```python
from build123d import *

# Parameters (mm, degrees)
SKETCH_1_W          = 60
SKETCH_1_H          = 45
EXTRUDE_1_DEPTH     = 30
SKETCH_3_W          = 35.871207779
SKETCH_3_H          = 20
CUT_EXTRUDE_3_DEPTH = 62.71805709
CHAMFER_1_SIZE      = 8


with BuildPart() as part:
    # Эскиз1 → Вытянуть1 (new body)
    with BuildSketch(Plane(origin=(0, 0, 0), x_dir=(1, 0, 0), z_dir=(0, 1, 0))):
        with Locations((-19.019063342, 0)):
            Rectangle(SKETCH_1_W, SKETCH_1_H)
    extrude(amount=EXTRUDE_1_DEPTH)

    # Эскиз3 → Вытянуть3 (cut, through all)
    with BuildSketch(Plane(origin=(0, 30, 0), x_dir=(1, 0, 0), z_dir=(0, 1, 0))):
        with Locations((-38.69487705, 0)):
            Rectangle(SKETCH_3_W, SKETCH_3_H)
    extrude(amount=-CUT_EXTRUDE_3_DEPTH, mode=Mode.SUBTRACT)

    # Фаска1
    chamfer_1_edges = [part.edges().sort_by_distance(p)[0] for p in [
        (-49.019063342, 30, -16.25),
        (-49.019063342, 0, 16.25),
        (-49.019063342, 30, 16.25),
        (-49.019063342, 0, -16.25),
    ]]
    chamfer(chamfer_1_edges, length=CHAMFER_1_SIZE)


solid = part.part
```
Check sheet for the modelled part. Datum: model origin and axes. Units: mm. A direction names the side the tool comes from. Coordinates: 2 decimals unless noted, no trailing zeros. Loops run counter-clockwise (first coordinate to the right, second up) from the corner with the lowest first, then second, coordinate; pieces in that order, holes last.
1) Sectioned sample at A-A (x = -26.5). Record the boundary of the cut face in (y, z).
2) Release check for a two-part mould opening along Z. For faces 1 (the face through (10.981, 15, 0)), 2 (the face through (-19, 15, -22.5)), 3 (the face through (-20.759, 15, 0)) record: released by +Z, released by -Z, zero draft, split by the parting line, or undercut.
3) Sectioned sample at D-D (y = 26.5). Record the boundary of the cut face in (x, z).
4) Access from +Z, -Z, +X, -X, +Y, -Y to the whole of each face (thin tool, end or side, straight path). Record for faces 4 (the face through (-49.019, 15, -16)), 5 (the face through (-35, 15, 10)).
5) Sectioned sample at B-B (y = 11). Record the boundary of the cut face in (x, z), and give its area (3 significant figures).
6) Material ranges on probe 1 along Z at (x, y) = (-24, 19.5); probe 2 along X at (y, z) = (14, -2); probe 3 along X at (y, z) = (6.5, 16), recorded low to high.
7) Sectioned sample at C-C (z = -16). Record the boundary of the cut face in (x, y), and give its area (3 significant figures).
8) Gauge pin test, flat end, axial feed: pin 1 (6 mm diameter, centred on y = 8.5, z = 3, fed in from -X). Record the tip position at first contact, or that the pin passes through.
Check sheet entries:
1. outline: (0, -22.5) - (30, -22.5) - (30, -10) - (0, -10) - close; (0, 10) - (30, 10) - (30, 22.5) - (0, 22.5) - close
2. face 1: zero draft
2. face 2: released by -Z
2. face 3: undercut
3. outline: (-44.52, -22.5) - (10.98, -22.5) - (10.98, 22.5) - (-44.52, 22.5) - (-44.52, 10) - (-20.76, 10) - (-20.76, -10) - (-44.52, -10) - close
4. face 4: +Z, -Z, -X, +Y, -Y
4. face 5: -X, +Y, -Y
5. outline: (-49.02, -22.5) - (10.98, -22.5) - (10.98, 22.5) - (-49.02, 22.5) - (-49.02, 10) - (-20.76, 10) - (-20.76, -10) - (-49.02, -10) - close
5. area: 2,130 mm2
6. probe 1: z = -22.5 to -10, 10 to 22.5
6. probe 2: x = -20.76 to 10.98
6. probe 3: x = -47.52 to 10.98
7. outline: (-49.02, 8) - (-41.02, 0) - (10.98, 0) - (10.98, 30) - (-41.02, 30) - (-49.02, 22) - close
7. area: 1,740 mm2
8. pin 1: stops at x = -20.76
